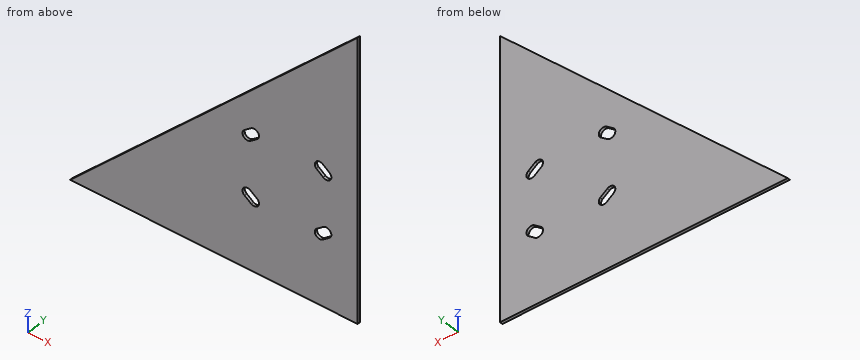
from build123d import *

# Parameters (mm, degrees)
BOSS_EXTRUDE1_DEPTH = 3.175


with BuildPart() as part:
    # Sketch1 → Boss-Extrude1 (new body)
    with BuildSketch(Plane(origin=(0, 0, 0), x_dir=(1, 0, 0), z_dir=(0, 1, 0))):
        Polygon((81.28, -209.55), (81.28, 120.65), (-248.92, 120.65), align=None)
        with BuildLine():
            Line((-48.781915156, 37.648908469), (-40.711239573, 43.820601562))
            ThreePointArc((-40.711239573, 43.820601562), (-33.204324417, 42.366693093), (-33.768084844, 34.741091531))
            Line((-33.768084844, 34.741091531), (-41.838760427, 28.569398438))
            ThreePointArc((-41.838760427, 28.569398438), (-49.850092807, 29.637576089), (-48.781915156, 37.648908469))
        make_face(mode=Mode.SUBTRACT)
        with BuildLine():
            Line((33.768084844, 34.741091531), (41.838760427, 28.569398438))
            ThreePointArc((41.838760427, 28.569398438), (49.850092807, 29.637576089), (48.781915156, 37.648908469))
            Line((48.781915156, 37.648908469), (40.711239573, 43.820601562))
            ThreePointArc((40.711239573, 43.820601562), (33.204324417, 42.366693093), (33.768084844, 34.741091531))
        make_face(mode=Mode.SUBTRACT)
        with BuildLine():
            Line((33.768084844, -34.741091531), (41.838760427, -28.569398438))
            ThreePointArc((41.838760427, -28.569398438), (49.850092807, -29.637576089), (48.781915156, -37.648908469))
            Line((48.781915156, -37.648908469), (40.711239573, -43.820601562))
            ThreePointArc((40.711239573, -43.820601562), (33.204324417, -42.366693093), (33.768084844, -34.741091531))
        make_face(mode=Mode.SUBTRACT)
        with BuildLine():
            Line((-48.781915156, -37.648908469), (-40.711239573, -43.820601562))
            ThreePointArc((-40.711239573, -43.820601562), (-33.204324417, -42.366693093), (-33.768084844, -34.741091531))
            Line((-33.768084844, -34.741091531), (-41.838760427, -28.569398438))
            ThreePointArc((-41.838760427, -28.569398438), (-49.850092807, -29.637576089), (-48.781915156, -37.648908469))
        make_face(mode=Mode.SUBTRACT)
    extrude(amount=BOSS_EXTRUDE1_DEPTH)


solid = part.part
Design review of the part built by this model. Coordinates are the model's own, in mm. Coordinates: 2 decimals unless noted, no trailing zeros. Order: outer loops, then holes, each group sorted by start corner. A loop starts at its lowest first (then second) coordinate and runs counter-clockwise, first axis right, second up.
Item 1: Take a section at A-A, the plane y = 1.8. Write out the cut boundary in (x, z) (3 decimals), then the cut area to 3 significant figures.
Item 2: Take a section at B-B, the plane z = 125. Write out the cut boundary in (x, y) (3 decimals).
Item 3: Take a section at C-C, the plane x = -227. Write out the cut boundary in (y, z) (3 decimals).
Item 4: For line 1 (X direction, y = 0.6, z = 44); line 2 (X direction, y = 2.1, z = 42); line 3 (Z direction, x = 43.5, y = 2.25), list the stretches that pass through material, from the lowest coordinate up.
The answers:
1. outline: (-248.92, -120.65) - (81.28, -120.65) - (81.28, 209.55) - close; hole (-48.782, -37.649) - (-40.711, -43.821) arc R5.755 ccw to (-33.768, -34.741) - (-41.839, -28.569) arc R5.715 ccw to start; hole (-48.782, 37.649) arc R5.715 ccw to (-41.839, 28.569) - (-33.768, 34.741) arc R5.755 ccw to (-40.711, 43.821) - close; hole (33.768, -34.741) arc R5.755 ccw to (40.711, -43.821) - (48.782, -37.649) arc R5.715 ccw to (41.839, -28.569) - close; hole (33.768, 34.741) - (41.839, 28.569) arc R5.715 ccw to (48.782, 37.649) - (40.711, 43.821) arc R5.755 ccw to start
1. area: 53,700 mm2
2. outline: (-3.27, 0) - (81.28, 0) - (81.28, 3.175) - (-3.27, 3.175) - close
3. outline: (0, -120.65) - (3.175, -120.65) - (3.175, -98.73) - (0, -98.73) - close
4. line 1: x = -84.27 to -40.39, -35.17 to 35.17, 40.39 to 81.28
4. line 2: x = -86.27 to -43.09, -32.95 to 32.95, 43.09 to 81.28
4. line 3: z = -120.65 to -41.69, -27.69 to 27.69, 41.69 to 171.77
